Design review of the part built by this model. Coordinates are the model's own, in mm. Face numbers are marked on the shaded views. A direction names the side the tool comes from. Coordinates: 2 decimals unless noted, no trailing zeros. Write each loop counter-clockwise with the first axis right and the second up, starting at its lowest first coordinate (ties: lowest second). Pieces come first, ordered by that corner, then holes. Notation, with made-up numbers: M 66,36.25 L 124,36.25 A23 ccw 124,64.25 Z; hole C -32.75,-21.75 d10. An arc over 180 degrees is marked long. Write item = value, one per line.
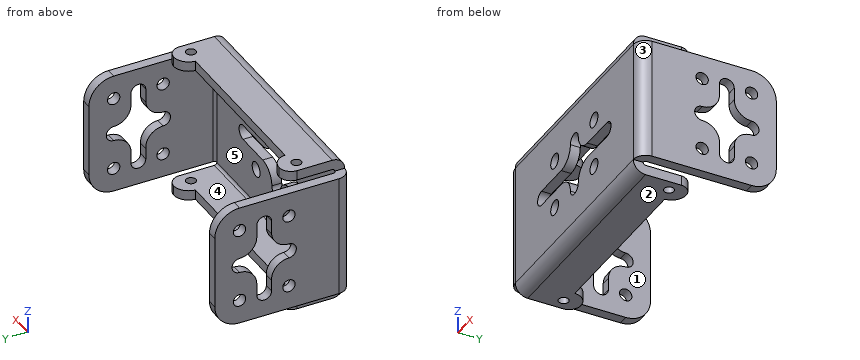
```python
from build123d import *

# Parameters (mm, degrees)
CROQUIS2_W             = 45
CROQUIS2_H             = 24.7
BRIDA_BASE1_DEPTH      = 2
BRIDA_DE_ARISTA1_DEPTH = 24.7
BRIDA_DE_ARISTA2_DEPTH = 24.7
BRIDA_DE_ARISTA3_DEPTH = 45
BRIDA_DE_ARISTA4_DEPTH = 45
CROQUIS34_R            = 1.25
CORTAR_EXTRUIR2_DEPTH  = 59.102345047
REDONDEO2_R            = 5
CROQUIS35_R            = 1
CORTAR_EXTRUIR3_DEPTH  = 47.502150488
CROQUIS36_R            = 1.5
CORTAR_EXTRUIR4_DEPTH  = 10


# Sheet-metal steps are written as plain solids
with BuildPart() as part:
    # Croquis2 → Brida base1 (new body)
    with BuildSketch(Plane(origin=(0, 0, 0), x_dir=(1, 0, 0), z_dir=(0, 1, 0))):
        Rectangle(CROQUIS2_W, CROQUIS2_H)
    extrude(amount=-BRIDA_BASE1_DEPTH)

    # Brida de arista1 section (across the edge) → Brida de arista1 (add)
    with BuildSketch(Plane(origin=(23, 0, 12.35), x_dir=(-1, 0, 0), z_dir=(0, 0, -1))):
        with BuildLine():
            Line((-2, 0.5), (-2, 25.6))
            Line((-2, 25.6), (0, 25.6))
            Line((0, 25.6), (0, 0.5))
            ThreePointArc((0, 0.5), (0.146446609, 0.146446609), (0.5, 0))
            Line((0.5, 0), (0.5, -2))
            ThreePointArc((0.5, -2), (-1.267766953, -1.267766953), (-2, 0.5))
        make_face()
    extrude(amount=BRIDA_DE_ARISTA1_DEPTH)

    # Brida de arista2 section (across the edge) → Brida de arista2 (add)
    with BuildSketch(Plane(origin=(-23, 0, -12.35), x_dir=(1, 0, 0), z_dir=(0, 0, 1))):
        with BuildLine():
            Line((-2, 0.5), (-2, 25.6))
            Line((-2, 25.6), (0, 25.6))
            Line((0, 25.6), (0, 0.5))
            ThreePointArc((0, 0.5), (0.146446609, 0.146446609), (0.5, 0))
            Line((0.5, 0), (0.5, -2))
            ThreePointArc((0.5, -2), (-1.267766953, -1.267766953), (-2, 0.5))
        make_face()
    extrude(amount=BRIDA_DE_ARISTA2_DEPTH)

    # Brida de arista3 section (across the edge) → Brida de arista3 (add)
    with BuildSketch(Plane(origin=(22.5, 0, -12.85), x_dir=(0, 0, 1), z_dir=(-1, 0, 0))):
        with BuildLine():
            Line((-2, 0.5), (-2, 10))
            Line((-2, 10), (0, 10))
            Line((0, 10), (0, 0.5))
            ThreePointArc((0, 0.5), (0.146446609, 0.146446609), (0.5, 0))
            Line((0.5, 0), (0.5, -2))
            ThreePointArc((0.5, -2), (-1.267766953, -1.267766953), (-2, 0.5))
        make_face()
    extrude(amount=BRIDA_DE_ARISTA3_DEPTH)

    # Brida de arista4 section (across the edge) → Brida de arista4 (add)
    with BuildSketch(Plane(origin=(-22.5, 0, 12.85), x_dir=(0, 0, -1), z_dir=(1, 0, 0))):
        with BuildLine():
            Line((-2, 0.5), (-2, 10))
            Line((-2, 10), (0, 10))
            Line((0, 10), (0, 0.5))
            ThreePointArc((0, 0.5), (0.146446609, 0.146446609), (0.5, 0))
            Line((0.5, 0), (0.5, -2))
            ThreePointArc((0.5, -2), (-1.267766953, -1.267766953), (-2, 0.5))
        make_face()
    extrude(amount=BRIDA_DE_ARISTA4_DEPTH)

    # Croquis34 → Cortar-Extruir2 (cut, through all)
    with BuildSketch(Plane.ZY.offset(25)):
        with Locations(Location((-7.5, 20.6, 0), (0, 0, 270))):
            Circle(CROQUIS34_R)
        with Locations(Location((7.5, 20.6, 0), (0, 0, 270))):
            Circle(CROQUIS34_R)
        with Locations(Location((7.5, 10.6, 0), (0, 0, 270))):
            Circle(CROQUIS34_R)
        with Locations(Location((-7.5, 10.6, 0), (0, 0, 270))):
            Circle(CROQUIS34_R)
        with BuildLine():
            Line((-7.5, 17.1), (-5, 17.1))
            ThreePointArc((-5, 17.1), (-2.525126266, 18.125126266), (-1.5, 20.6))
            ThreePointArc((-1.5, 20.6), (0, 22.1), (1.5, 20.6))
            ThreePointArc((1.5, 20.6), (2.525126266, 18.125126266), (5, 17.1))
            Line((5, 17.1), (7.5, 17.1))
            ThreePointArc((7.5, 17.1), (9, 15.6), (7.5, 14.1))
            Line((7.5, 14.1), (4.704458788, 14.1))
            ThreePointArc((4.704458788, 14.1), (2.422114194, 12.972686037), (1.5, 10.6))
            ThreePointArc((1.5, 10.6), (0, 9.1), (-1.5, 10.6))
            ThreePointArc((-1.5, 10.6), (-2.631035123, 13.181478893), (-5.295541212, 14.1))
            Line((-5.295541212, 14.1), (-7.5, 14.1))
            ThreePointArc((-7.5, 14.1), (-9, 15.6), (-7.5, 17.1))
        make_face()
    extrude(amount=-CORTAR_EXTRUIR2_DEPTH, mode=Mode.SUBTRACT)

    # Redondeo2
    redondeo2_edges = [part.edges().sort_by_distance(p)[0] for p in [
        (24, 25.6, 12.35),
        (24, 25.6, -12.35),
        (-24, 25.6, -12.35),
        (-24, 25.6, 12.35),
    ]]
    fillet(redondeo2_edges, radius=REDONDEO2_R)

    # Croquis35 → Cortar-Extruir3 (cut, through all)
    with BuildSketch(Plane.XY.offset(14.85)):
        with BuildLine():
            ThreePointArc((-22.5, 7.6), (-21.797056275, 9.297056275), (-20.1, 10))
            Line((-20.1, 10), (-22.5, 10))
            Line((-22.5, 10), (-22.5, 7.6))
        make_face()
        with BuildLine():
            ThreePointArc((-20.1, 10), (-18.050609847, 9.19089023), (-17.106674091, 7.2))
            Line((-17.106674091, 7.2), (17.106674091, 7.2))
            ThreePointArc((17.106674091, 7.2), (18.050609847, 9.19089023), (20.1, 10))
            Line((20.1, 10), (-20.1, 10))
        make_face()
        with BuildLine():
            Line((22.5, 10), (20.1, 10))
            ThreePointArc((20.1, 10), (21.750190132, 9.344164297), (22.5, 7.734495665))
            Line((22.5, 7.734495665), (22.5, 10))
        make_face()
        with Locations((-20.1, 6.5)):
            Circle(CROQUIS35_R)
        with Locations((20.1, 6.5)):
            Circle(CROQUIS35_R)
    extrude(amount=-CORTAR_EXTRUIR3_DEPTH, mode=Mode.SUBTRACT)

    # Croquis36 → Cortar-Extruir4 (cut)
    with BuildSketch(Plane.XZ.offset(2)):
        with BuildLine():
            Line((-5, 1.5), (-12.5, 1.5))
            ThreePointArc((-12.5, 1.5), (-14, 0), (-12.5, -1.5))
            Line((-12.5, -1.5), (-5, -1.5))
            ThreePointArc((-5, -1.5), (-2.525126266, -2.525126266), (-1.5, -5))
            ThreePointArc((-1.5, -5), (0, -6.5), (1.5, -5))
            ThreePointArc((1.5, -5), (2.525126266, -2.525126266), (5, -1.5))
            Line((5, -1.5), (12.5, -1.5))
            ThreePointArc((12.5, -1.5), (14, 0), (12.5, 1.5))
            Line((12.5, 1.5), (5, 1.5))
            ThreePointArc((5, 1.5), (2.525126266, 2.525126266), (1.5, 5))
            ThreePointArc((1.5, 5), (0, 6.5), (-1.5, 5))
            ThreePointArc((-1.5, 5), (-2.525126266, 2.525126266), (-5, 1.5))
        make_face()
        with Locations(Location((-7.5, 5, 0), (0, 0, 270))):
            Circle(CROQUIS36_R)
        with Locations(Location((7.5, 5, 0), (0, 0, 270))):
            Circle(CROQUIS36_R)
        with Locations(Location((7.5, -5, 0), (0, 0, 270))):
            Circle(CROQUIS36_R)
        with Locations(Location((-7.5, -5, 0), (0, 0, 270))):
            Circle(CROQUIS36_R)
    extrude(amount=-CORTAR_EXTRUIR4_DEPTH, mode=Mode.SUBTRACT)


solid = part.part
```
Q1. For P1, Ø1.6, axis at x = -7.5, z = 14, coming from the +Y side; P2, Ø2, axis at y = 2, z = 14, coming from the +X side; P3, Ø3, axis at x = 23, y = 12, coming from the +Z side; P4, Ø10, axis at x = -2, y = 14.5, coming from the +Z side, all flat-tipped, find the tip position at first contact; note any pin that passes through.
Check result:
P1 = 7.2
P2 = 22.5
P3 = 12.35
P4 = through
Q2. Machinability: for the marked faces 1 and 2, which of the approach directions +Z, -Z, +X, -X, +Y, -Y give a long, thin tool a straight path to every point of the face, cutting with its end or side? Answer none if there is none.
Check result:
face_1 = +Z, -Z, +Y
face_2 = -Z, +X, -X, +Y, -Y
Q3. Consider section C-C, the plane z = 0. State the section outline as (x, y) points.
Check result:
outline = M -25,0.5 A2.5 ccw -22.5,-2 L -14,-2 L -14,0 L -22.5,0 A0.5 cw -23,0.5 L -23,9.1 L -25,9.1 Z; M -25,22.1 L -23,22.1 L -23,25.6 L -25,25.6 Z; M 14,-2 L 22.5,-2 A2.5 ccw 25,0.5 L 25,9.1 L 23,9.1 L 23,0.5 A0.5 cw 22.5,0 L 14,0 Z; M 23,22.1 L 25,22.1 L 25,25.6 L 23,25.6 Z
Q4. Consider section D-D, the plane x = 7.5. State the section outline as (y, z) points.
Check result:
outline = M -2,-12.35 A2.5 ccw 0.5,-14.85 L 7.2,-14.85 L 7.2,-12.85 L 0.5,-12.85 A0.5 cw 0,-12.35 L 0,-6.5 L -2,-6.5 Z; M -2,-3.5 L 0,-3.5 L 0,-1.5 L -2,-1.5 Z; M -2,1.5 L 0,1.5 L 0,3.5 L -2,3.5 Z; M -2,6.5 L 0,6.5 L 0,12.35 A0.5 cw 0.5,12.85 L 7.2,12.85 L 7.2,14.85 L 0.5,14.85 A2.5 ccw -2,12.35 Z
Q5. The part is to be moulded in two halves that separate along X. For the marked faces 3, 4 and 5, say which applies: +X half, -X half, draft (parallel to the pull), parting line (faces both ways), or undercut.
Check result:
face_3 = +X half
face_4 = draft
face_5 = undercut
Q6. Wall thickness on line 1 (Z direction, x = -24.4, y = 20.6); line 2 (X direction, y = 3.5, z = -7.5); line 3 (Z direction, x = -14, y = 5.25): over which ranges is each line inside the solid? List them lowest first.
Check result:
line_1 = -12.35 to -8.75, -6.25 to -1.5, 1.5 to 6.25, 8.75 to 12.35
line_2 = -25 to -23, 23 to 25
line_3 = -14.85 to -12.85, 12.85 to 14.85
Q7. Consider section A-A, the plane x = 0. State the section outline as (y, z) points, and give its area (3 significant figures).
Check result:
outline = M -2,-12.35 A2.5 ccw 0.5,-14.85 L 7.2,-14.85 L 7.2,-12.85 L 0.5,-12.85 A0.5 cw 0,-12.35 L 0,-6.5 L -2,-6.5 Z; M -2,6.5 L 0,6.5 L 0,12.35 A0.5 cw 0.5,12.85 L 7.2,12.85 L 7.2,14.85 L 0.5,14.85 A2.5 ccw -2,12.35 Z
area = 59.6 mm²
Q8. Consider section B-B, the plane y = 4.5. State the section outline as (x, z) points, and give its area (3 significant figures).
Check result:
outline = M -25,-12.35 L -23,-12.35 L -23,12.35 L -25,12.35 Z; M -22.5,-14.85 L 22.5,-14.85 L 22.5,-12.85 L -22.5,-12.85 Z; M -22.5,12.85 L 22.5,12.85 L 22.5,14.85 L -22.5,14.85 Z; M 23,-12.35 L 25,-12.35 L 25,12.35 L 23,12.35 Z
area = 279 mm²
